```python
from build123d import *

# Parameters (mm, degrees)
SKETCH1_W           = 22
SKETCH1_H           = 12
BOSS_EXTRUDE1_DEPTH = 15
SKETCH2_W           = 32
SKETCH2_H           = 12
BOSS_EXTRUDE2_DEPTH = 2
SKETCH4_W           = 22
SKETCH4_H           = 12
BOSS_EXTRUDE3_DEPTH = 2
SKETCH5_R           = 6
BOSS_EXTRUDE4_DEPTH = 4
SKETCH6_R           = 3.5
BOSS_EXTRUDE5_DEPTH = 5
BOSS_EXTRUDE6_START = -2
BOSS_EXTRUDE6_DEPTH = 2
CUT_EXTRUDE1_REACH  = 29.797
SKETCH8_R           = 0.75


with BuildPart() as part:
    # Sketch1 → Boss-Extrude1 (new body)
    with BuildSketch(Plane(origin=(0, 0, 0), x_dir=(1, 0, 0), z_dir=(0, 1, 0))):
        Rectangle(SKETCH1_W, SKETCH1_H)
    extrude(amount=BOSS_EXTRUDE1_DEPTH)

    # Sketch2 → Boss-Extrude2 (add)
    with BuildSketch(Plane(origin=(0, 15, 0), x_dir=(1, 0, 0), z_dir=(0, 1, 0))):
        Rectangle(SKETCH2_W, SKETCH2_H)
    extrude(amount=BOSS_EXTRUDE2_DEPTH)

    # Sketch4 → Boss-Extrude3 (add)
    with BuildSketch(Plane(origin=(0, 17, 0), x_dir=(1, 0, 0), z_dir=(0, 1, 0))):
        Rectangle(SKETCH4_W, SKETCH4_H)
    extrude(amount=BOSS_EXTRUDE3_DEPTH)

    # Sketch5 → Boss-Extrude4 (add)
    with BuildSketch(Plane(origin=(0, 19, 0), x_dir=(1, 0, 0), z_dir=(0, 1, 0))):
        with Locations(Location((-5, 0, 0), (0, 0, 270))):
            Circle(SKETCH5_R)
    extrude(amount=BOSS_EXTRUDE4_DEPTH)

    # Sketch6 → Boss-Extrude5 (add)
    with BuildSketch(Plane(origin=(0, 23, 0), x_dir=(1, 0, 0), z_dir=(0, 1, 0))):
        with Locations(Location((-5, 0, 0), (0, 0, 270))):
            Circle(SKETCH6_R)
    extrude(amount=BOSS_EXTRUDE5_DEPTH)

    # Sketch7 → Boss-Extrude6 (add)
    with BuildSketch(Plane(origin=(0, 28, 0), x_dir=(1, 0, 0), z_dir=(0, 1, 0)).offset(BOSS_EXTRUDE6_START)):
        with BuildLine():
            Line((-17.394274369, 9.57939802), (-7.704984199, -2.22104941))
            ThreePointArc((-7.704984199, -2.22104941), (-7.474873734, 2.474873734), (-2.77895059, 2.704984199))
            Line((-2.77895059, 2.704984199), (-14.57939802, 12.394274369))
            ThreePointArc((-14.57939802, 12.394274369), (-17.262782674, 12.262782674), (-17.394274369, 9.57939802))
        make_face()
    extrude(amount=BOSS_EXTRUDE6_DEPTH)

    # Sketch8 → Cut-Extrude1 (cut, up to next)
    with BuildSketch(Plane(origin=(0, 17, 0), x_dir=(1, 0, 0), z_dir=(0, 1, 0)), mode=Mode.PRIVATE) as cut_extrude1_sk1:
        with Locations(Location((13.5, 0, 0), (0, 0, 270))):
            Circle(SKETCH8_R)
    cut_extrude1_tool1 = extrude(cut_extrude1_sk1.sketch, amount=-CUT_EXTRUDE1_REACH, mode=Mode.PRIVATE) & part.part
    # Sketch8 → Cut-Extrude1 (cut, up to next)
    with BuildSketch(Plane(origin=(0, 17, 0), x_dir=(1, 0, 0), z_dir=(0, 1, 0)), mode=Mode.PRIVATE) as cut_extrude1_sk2:
        with Locations(Location((-13.5, 0, 0), (0, 0, 270))):
            Circle(SKETCH8_R)
    cut_extrude1_tool2 = extrude(cut_extrude1_sk2.sketch, amount=-CUT_EXTRUDE1_REACH, mode=Mode.PRIVATE) & part.part
    add(cut_extrude1_tool1.solids().sort_by_distance((13.5, 17, 0))[0], mode=Mode.SUBTRACT)
    add(cut_extrude1_tool2.solids().sort_by_distance((-13.5, 17, 0))[0], mode=Mode.SUBTRACT)


solid = part.part
```
The model under review builds one solid part; all positions refer to its coordinate system, in mm. A direction names the side the tool comes from. Round coordinates to 2 decimals unless told otherwise and drop trailing zeros. Loops run counter-clockwise (first coordinate to the right, second up) from the corner with the lowest first, then second, coordinate; pieces in that order, holes last. Notation, with made-up numbers: (-5, 65.25) -> (51, 65.25) arc R6 ccw to (51, 69.25) -> close; hole circle Ø8 at (-21, 83). An arc over 180 degrees is marked (long way). Answer in a Markdown table with one row per item.
1) Consider section A-A, the plane x = 13.5. Write out the cut boundary in (y, z), plus the area to 3 significant figures.
Taken from the geometry:
| item | result |
|---|---|
| outline | (15, -6) -> (17, -6) -> (17, -0.75) -> (15, -0.75) -> close; (15, 0.75) -> (17, 0.75) -> (17, 6) -> (15, 6) -> close |
| area | 21.0 mm² |
2) Consider section D-D, the plane y = 20. Write out the cut boundary in (x, z).
Taken from the geometry:
| item | result |
|---|---|
| outline | circle Ø12 at (-5, 0) |
3) For pin 1 Ø5.5 at (x, z) = (-14, 1.5) entering from +Y; pin 2 Ø1.5 at (x, z) = (-12.5, 1) entering from -Y; pin 3 Ø5 at (x, z) = (2.5, -8) entering from +Y, all flat-tipped, find the tip position at first contact; note any pin that passes through.
Taken from the geometry:
| item | result |
|---|---|
| pin 1 | stops at y = 17 |
| pin 2 | stops at y = 15 |
| pin 3 | stops at y = 19 |
4) Draft analysis for pull direction Y (two halves, no side actions). For faces 1 (the flat face through (-11, 26, -7)), 2 (the flat face through (5, 19, 0)), 3 (the flat face through (11, 7, 0)), state which applies: pulls with the +Y half, pulls with the -Y half, needs draft (parallel to the pull), parting line crosses it, or undercut.
Taken from the geometry:
| item | result |
|---|---|
| face 1 | undercut |
| face 2 | pulls with the +Y half |
| face 3 | needs draft |
5) Consider section B-B, the plane x = -13.5. Write out the cut boundary in (y, z).
Taken from the geometry:
| item | result |
|---|---|
| outline | (15, -6) -> (17, -6) -> (17, -0.75) -> (15, -0.75) -> close; (15, 0.75) -> (17, 0.75) -> (17, 6) -> (15, 6) -> close; (26, -11.51) -> (28, -11.51) -> (28, -4.84) -> (26, -4.84) -> close |
6) Wall thickness on line 1 along X through (y, z) = (15.7, 0); line 2 along Z through (x, y) = (-7, 9.5); line 3 along X through (y, z) = (17.25, 0.5): over which ranges is each line inside the solid? List them lowest first.
Taken from the geometry:
| item | result |
|---|---|
| line 1 | x = -16 to -14.25, -12.75 to 12.75, 14.25 to 16 |
| line 2 | z = -6 to 6 |
| line 3 | x = -11 to 11 |
7) Tool access review of faces 4 (the flat face through (-12.617, 26.986, -3.762)), 5 (the flat face through (11, 18, 0)), 6 (the flat face through (-12, 15, 0)), 7 (the flat face through (-10, 19, -5)), 8 (the flat face through (0, 9, -6)): name each direction out of +Z, -Z, +X, -X, +Y, -Y from which nothing blocks a thin tool from reaching the whole face with its end or side.
Taken from the geometry:
| item | result |
|---|---|
| face 4 | +Z, -X, +Y |
| face 5 | +Z, -Z, +X, +Y |
| face 6 | +Z, -Z, -X, -Y |
| face 7 | -Z, -X |
| face 8 | -Z, +X, -X, -Y |
8) Consider section C-C, the plane x = 6. Write out the cut boundary in (y, z).
Taken from the geometry:
| item | result |
|---|---|
| outline | (0, -6) -> (19, -6) -> (19, 6) -> (0, 6) -> close |
